Check sheet for the modelled part. Datum: model origin and axes. Units: mm. A direction names the side the tool comes from. Coordinates: 2 decimals unless noted, no trailing zeros. Loops run counter-clockwise (first coordinate to the right, second up) from the corner with the lowest first, then second, coordinate; pieces in that order, holes last. Notation, with made-up numbers: (28.25, -8.5) -> (40.25, -8.5) arc R21 cw to (40.25, 3.5) -> close; hole circle Ø4 at (-31.5, -20.75). An arc over 180 degrees is marked (long way). Use one line per item in the form item = value.
from build123d import *

# Parameters (mm, degrees)
F0_W     = 23.6952770501
F0_H     = 60.1157741621
F1_DEPTH = 75
F2_R     = 16.1345340931
F3_DEPTH = 23.6962770501
F4_R     = 6.5
F5_DEPTH = 23.6962658743
F6_R     = 5


with BuildPart() as f1:
    # F0 (on Front) → F1 (new body)
    with BuildSketch(Plane.XZ):
        Polygon((-42.5637289882, -11.8476329371), (42.5637289882, -11.8476329371), (42.5637289882, 11.8476329371), (-18.868451938, 11.8476329371), (-42.5637289882, 11.8476329371), align=None)
        with Locations((-30.7160904631, 41.9055200182)):
            Rectangle(F0_W, F0_H)
    extrude(amount=-F1_DEPTH)

    # F2 (on face) → F3 (cut, through all)
    with BuildSketch(Plane.YZ.offset(-18.868451938)):
        with Locations((37.5, 41.9055200182)):
            Circle(F2_R)
    extrude(amount=-F3_DEPTH, mode=Mode.SUBTRACT)

    # F4 (on face) → F5 (cut, through all)
    with BuildSketch(Plane.XY.offset(11.8476329371)):
        with Locations((11.8476385251, 20.3867554665)):
            Circle(F4_R)
        with Locations((11.8476385251, 50.6640449166)):
            Circle(F4_R)
    extrude(amount=-F5_DEPTH, mode=Mode.SUBTRACT)

    # F6
    f6_edges = [f1.edges().sort_by_distance(p)[0] for p in [
        (-30.71609, 0, 71.963407),
        (-30.71609, 75, 71.963407),
    ]]
    fillet(f6_edges, radius=F6_R)


solid = f1.part
(1) Go/stop test with a flat-tipped pin: P1, Ø3, axis at x = -6.5, y = 22.5, coming from the +Z side. Record where the tip stops, or that it passes through.
Established:
P1 = 11.85
(2) Section check C-C, the plane y = 46. Record the boundary of the cut face in (x, z), plus the area to 3 significant figures.
Established:
outline = (-42.56, -11.85) -> (7.32, -11.85) -> (7.32, 11.85) -> (-18.87, 11.85) -> (-18.87, 28.19) -> (-42.56, 28.19) -> close; (-42.56, 55.62) -> (-18.87, 55.62) -> (-18.87, 71.96) -> (-42.56, 71.96) -> close; (16.37, -11.85) -> (42.56, -11.85) -> (42.56, 11.85) -> (16.37, 11.85) -> close
area = 2,580 mm²
(3) Section check B-B, the plane z = 40.5. Record the boundary of the cut face in (x, y).
Established:
outline = (-42.56, 0) -> (-18.87, 0) -> (-18.87, 21.43) -> (-42.56, 21.43) -> close; (-42.56, 53.57) -> (-18.87, 53.57) -> (-18.87, 75) -> (-42.56, 75) -> close
(4) Mould release check, pull along X, two halves, no side actions. Record for faces 1 (the cylindrical face through (18.047, 22.339, 0.166)), 2 (the flat face through (42.564, 37, 0)), 3 (the flat face through (-42.564, 37, 21)): +X half, -X half, draft (parallel to the pull), parting line (faces both ways), or undercut.
Established:
face_1 = undercut
face_2 = +X half
face_3 = -X half
(5) Scan lines: line 1 along Y through (x, z) = (6, -2); line 2 along X through (y, z) = (15, 56); line 3 along Z through (x, y) = (-4.5, 57). Record each from-to range of solid material in increasing order.
Established:
line_1 = 0 to 17.55, 23.22 to 47.83, 53.5 to 75
line_2 = -42.56 to -18.87
line_3 = -11.85 to 11.85
(6) Section check A-A, the plane y = 37.5. Record the boundary of the cut face in (x, z), plus the area to 3 significant figures.
Established:
outline = (-42.56, -11.85) -> (42.56, -11.85) -> (42.56, 11.85) -> (-18.87, 11.85) -> (-18.87, 25.77) -> (-42.56, 25.77) -> close; (-42.56, 58.04) -> (-18.87, 58.04) -> (-18.87, 71.96) -> (-42.56, 71.96) -> close
area = 2,680 mm²
(7) Tool access check on faces 4 (the cylindrical face through (-30.55, 1.426, 70.46)), 5 (the flat face through (-18.868, 29, 28)). Record the directions out of +Z, -Z, +X, -X, +Y, -Y that give a thin tool (end or side, any length) a straight path to the whole face; none if there is none.
Established:
face_4 = +Z, +X, -X, -Y
face_5 = +Z, +X, +Y, -Y
(8) Section check D-D, the plane x = -33.5. Record the boundary of the cut face in (y, z), plus the area to 3 significant figures.
Established:
outline = (0, -11.85) -> (75, -11.85) -> (75, 66.96) arc R5 ccw to (70, 71.96) -> (5, 71.96) arc R5 ccw to (0, 66.96) -> close; hole circle Ø32.27 at (37.5, 41.91)
area = 5,460 mm²
